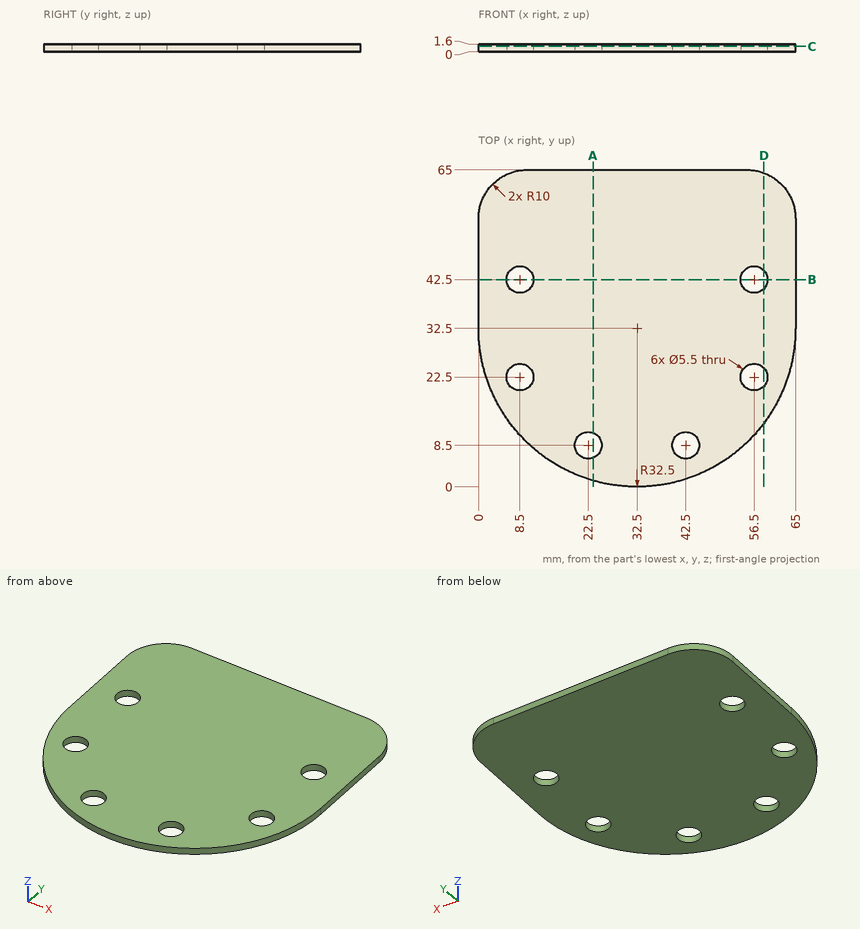
Job drawing, mm, ordinate dimensions from the low corner. One solid piece. Round coordinates to 2 decimals unless told otherwise and drop trailing zeros. Order: outer loops, then holes, each group sorted by start corner. A loop starts at its lowest first (then second) coordinate and runs counter-clockwise, first axis right, second up. Notation, with made-up numbers: M 37.5,0.5 L 95.5,0.5 A15 cw 95.5,13.5 Z; hole C -9.5,36.25 d11. An arc over 180 degrees is marked long. Write each question's results on one line, items separated by ' | '. Start each with the question number.
(1) Saw through at B-B, the plane y = 42.5. Give the cut face in (x, z).
(2) Saw through at A-A, the plane x = 23.5. Give the cut face in (y, z).
(3) Drop flat-ended pins along their axis: pin 1 (5 mm diameter, centred on x = 22.5, y = 8.5, fed in from +Z); pin 2 (7 mm diameter, centred on x = 8.5, y = 22.5, fed in from +Z). Give the stop position or say it passes through.
(4) Saw through at C-C, the plane z = 1.1. Give the cut face in (x, y), then the cut area to 3 significant figures.
(5) Saw through at D-D, the plane x = 58.5. Give the cut face in (y, z).
(6) Probe probe 1 along X at (y, z) = (20, 0.6) (1 decimal); probe 2 along X at (y, z) = (40, 0.9) (1 decimal); probe 3 along Y at (x, z) = (24, 0.15) (1 decimal). List the from-to ranges inside material, lowest first. Write a range as from..to.
Established:
1) outline: M 0,0 L 5.75,0 L 5.75,1.6 L 0,1.6 Z; M 11.25,0 L 53.75,0 L 53.75,1.6 L 11.25,1.6 Z; M 59.25,0 L 65,0 L 65,1.6 L 59.25,1.6 Z
2) outline: M 1.27,0 L 5.94,0 L 5.94,1.6 L 1.27,1.6 Z; M 11.06,0 L 65,0 L 65,1.6 L 11.06,1.6 Z
3) pin 1: passes through | pin 2: stops at z = 1.6
4) outline: M 0,32.5 A32.5 ccw 65,32.5 L 65,55 A10 ccw 55,65 L 10,65 A10 ccw 0,55 Z; hole C 8.5,22.5 d5.5; hole C 8.5,42.5 d5.5; hole C 22.5,8.5 d5.5; hole C 42.5,8.5 d5.5; hole C 56.5,22.5 d5.5; hole C 56.5,42.5 d5.5 | area: 3,590 mm^2
5) outline: M 13,0 L 20.61,0 L 20.61,1.6 L 13,1.6 Z; M 24.39,0 L 40.61,0 L 40.61,1.6 L 24.39,1.6 Z; M 44.39,0 L 64.37,0 L 64.37,1.6 L 44.39,1.6 Z
6) probe 1: x = 2.5..7.4, 9.6..55.4, 57.6..62.5 | probe 2: x = 0..7.4, 9.6..55.4, 57.6..65 | probe 3: y = 1.1..6.2, 10.8..65
